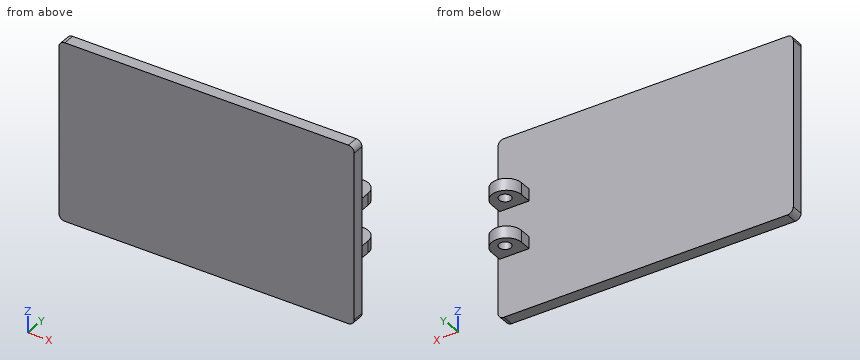
```python
from build123d import *

# Parameters (mm, degrees)
SKETCH1_W           = 500
SKETCH1_H           = 300
BOSS_EXTRUDE1_DEPTH = 20
BOSS_EXTRUDE2_START = -100
BOSS_EXTRUDE2_DEPTH = 20
SKETCH3_R           = 10
CUT_EXTRUDE1_DEPTH  = 286
FILLET1_R           = 10


with BuildPart() as part:
    # Sketch1 → Boss-Extrude1 (new body)
    with BuildSketch(Plane(origin=(0, 0, 0), x_dir=(1, 0, 0), z_dir=(0, 1, 0))):
        Rectangle(SKETCH1_W, SKETCH1_H)
    extrude(amount=BOSS_EXTRUDE1_DEPTH)

    # Sketch2 → Boss-Extrude2 (add)
    with BuildSketch(Plane.XY.offset(150).offset(BOSS_EXTRUDE2_START)):
        with BuildLine():
            Line((197.091467049, 40), (197.091467049, 0))
            Line((197.091467049, 0), (247.091467049, 0))
            Line((247.091467049, 0), (247.091467049, 40))
            ThreePointArc((247.091467049, 40), (222.091467049, 65), (197.091467049, 40))
        make_face()
    boss_extrude2 = extrude(amount=-BOSS_EXTRUDE2_DEPTH)

    # Mirror1: Boss-Extrude2 across plane
    add(boss_extrude2.mirror(Plane.XY))

    # Sketch3 → Cut-Extrude1 (cut)
    with BuildSketch(Plane.XY.offset(50)):
        with Locations(Location((221.220080181, 45.121109354, 0), (0, 0, 180))):
            Circle(SKETCH3_R)
    extrude(amount=-CUT_EXTRUDE1_DEPTH, mode=Mode.SUBTRACT)

    # Fillet1
    fillet1_edges = [part.edges().sort_by_distance(p)[0] for p in [
        (250, 10, 150),
        (-250, 10, 150),
        (-250, 10, -150),
        (250, 10, -150),
    ]]
    fillet(fillet1_edges, radius=FILLET1_R)


solid = part.part
```
For this review, take the finished solid that the model builds, in its own axes (mm). Round coordinates to 2 decimals unless told otherwise and drop trailing zeros. Order: outer loops, then holes, each group sorted by start corner. A loop starts at its lowest first (then second) coordinate and runs counter-clockwise, first axis right, second up.
Q1. We need section C-C, the plane x = 2. Give the boundary of the cut face in (y, z), plus the area to 3 significant figures.
Findings below:
outline: (0, -150) - (20, -150) - (20, 150) - (0, 150) - close
area: 6,000 mm2
Q2. We need section B-B, the plane z = 106. Give the boundary of the cut face in (x, y).
Findings below:
outline: (-250, 0) - (250, 0) - (250, 20) - (-250, 20) - close
Q3. We need section A-A, the plane y = 50. Give the boundary of the cut face in (x, z).
Findings below:
outline: (199.18, -50) - (212.49, -50) - (212.49, -30) - (199.18, -30) - close; (199.18, 30) - (212.49, 30) - (212.49, 50) - (199.18, 50) - close; (229.95, -50) - (245, -50) - (245, -30) - (229.95, -30) - close; (229.95, 30) - (245, 30) - (245, 50) - (229.95, 50) - close
Q4. Insertion check: P1, Ø10, axis at y = 26, z = 37, coming from the -X side; P2, Ø23, axis at x = 221.22, y = 45.12, coming from the +Z side; P3, Ø12, axis at x = 221.22, y = 45.12, coming from the -Z side; P4, Ø4, axis at x = -139.5, z = -25, coming from the +Y side. Each pin has a flat end and moves straight along its axis. Give the tip position at first contact, or say it passes through.
Findings below:
P1: stops at x = 197.09
P2: stops at z = 50
P3: passes through
P4: stops at y = 20
Q5. Wall thickness on line 1 (Y direction, x = -176.5, z = 28.5): over which ranges is the line inside the solid? List them lowest first.
Findings below:
line 1: y = 0 to 20
